from build123d import *

# Parameters (mm, degrees)
SKETCH1_R                = 17.45
SKETCH1_R_2              = 12.45
BOSS_EXTRUDE1_DEPTH      = 8
BOSS_EXTRUDE1_DEPTH_BACK = 25
SKETCH1_2_R              = 17.45
SKETCH1_2_R_2            = 12.45
BOSS_EXTRUDE3_DEPTH      = 18
SKETCH3_R                = 12.45
SKETCH3_R_2              = 8
BOSS_EXTRUDE4_DEPTH      = 3
SKETCH4_R                = 1
CUT_EXTRUDE1_DEPTH       = 10
SKETCH6_R                = 13.5
CUT_EXTRUDE2_DEPTH       = 40
SKETCH7_R                = 1
CUT_EXTRUDE3_DEPTH       = 21
CIRPATTERN1_COUNT        = 3
BOSS_EXTRUDE5_START      = -16.1
SKETCH8_R                = 20.25
SKETCH8_R_2              = 13.5
BOSS_EXTRUDE5_DEPTH      = 3
FILLET1_R                = 2
SKETCH9_W                = 226.458017819
SKETCH9_H                = 42.937005292
CUT_EXTRUDE4_DEPTH       = 34
CUT_EXTRUDE4_DEPTH_BACK  = 62
CUT_EXTRUDE5_START       = -1.9
CUT_EXTRUDE5_DEPTH       = 1.7
CUT_EXTRUDE5_DEPTH_BACK  = 1.3
SKETCH11_R               = 1
CUT_EXTRUDE6_DEPTH       = 3
CUT_EXTRUDE7_START       = -1.9
CUT_EXTRUDE7_DEPTH       = 1.7
SKETCH14_R               = 20.25
SKETCH14_R_2             = 1
SKETCH14_R_3             = 13.5
BOSS_EXTRUDE6_DEPTH      = 0.8


with BuildPart() as part:
    # Sketch1 → Boss-Extrude1 (new body, two sides)
    with BuildSketch(Plane(origin=(0, 0, 0), x_dir=(1, 0, 0), z_dir=(0, 1, 0))) as boss_extrude1_sk:
        Circle(SKETCH1_R)
        Circle(SKETCH1_R_2, mode=Mode.SUBTRACT)
    extrude(amount=BOSS_EXTRUDE1_DEPTH)
    extrude(boss_extrude1_sk.sketch, amount=-BOSS_EXTRUDE1_DEPTH_BACK)

    # Sketch1<2> → Boss-Extrude3 (add)
    with BuildSketch(Plane(origin=(0, 0, 0), x_dir=(1, 0, 0), z_dir=(0, 1, 0))):
        Circle(SKETCH1_2_R)
        Circle(SKETCH1_2_R_2, mode=Mode.SUBTRACT)
    extrude(amount=BOSS_EXTRUDE3_DEPTH)

    # Sketch3 → Boss-Extrude4 (add)
    with BuildSketch(Plane(origin=(0, 18, 0), x_dir=(1, 0, 0), z_dir=(0, 1, 0))):
        Circle(SKETCH3_R)
        Circle(SKETCH3_R_2, mode=Mode.SUBTRACT)
    extrude(amount=-BOSS_EXTRUDE4_DEPTH)

    # Sketch4 → Cut-Extrude1 (cut)
    with BuildSketch(Plane(origin=(0, 18, 0), x_dir=(1, 0, 0), z_dir=(0, 1, 0))):
        with Locations((9.526279442, 5.5)):
            Circle(SKETCH4_R)
        with Locations((-9.526279442, 5.5)):
            Circle(SKETCH4_R)
        with Locations((0, -11)):
            Circle(SKETCH4_R)
    extrude(amount=-CUT_EXTRUDE1_DEPTH, mode=Mode.SUBTRACT)

    # Sketch6 → Cut-Extrude2 (cut)
    with BuildSketch(Plane.XZ.offset(25)):
        Circle(SKETCH6_R)
    extrude(amount=-CUT_EXTRUDE2_DEPTH, mode=Mode.SUBTRACT)

    # Sketch7 → Cut-Extrude3 (cut)
    with BuildSketch(Plane.XY):
        with Locations((0, 12)):
            Circle(SKETCH7_R)
    cut_extrude3 = extrude(amount=-CUT_EXTRUDE3_DEPTH, mode=Mode.SUBTRACT)

    # CirPattern1: Cut-Extrude3 ×3 about axis
    cirpattern1_axis = Axis((0, 53.183766184, 0), (0, -1, 0))
    for i in range(1, CIRPATTERN1_COUNT):
        add(cut_extrude3.rotate(cirpattern1_axis, i * 360 / CIRPATTERN1_COUNT), mode=Mode.SUBTRACT)

    # Sketch8 → Boss-Extrude5 (add)
    with BuildSketch(Plane(origin=(0, 18, 0), x_dir=(1, 0, 0), z_dir=(0, 1, 0)).offset(BOSS_EXTRUDE5_START)):
        Circle(SKETCH8_R)
        Circle(SKETCH8_R_2, mode=Mode.SUBTRACT)
    extrude(amount=-BOSS_EXTRUDE5_DEPTH)

    # Fillet1
    fillet1_edges = [part.edges().sort_by_distance(p)[0] for p in [
        (-17.45, 18, 0),
    ]]
    fillet(fillet1_edges, radius=FILLET1_R)

    # Sketch9 → Cut-Extrude4 (cut, two sides)
    with BuildSketch(Plane(origin=(0, 0, 0), x_dir=(0, 0, -1), z_dir=(1, 0, 0))) as cut_extrude4_sk:
        with Locations((-4.854722567, -21.468502646)):
            Rectangle(SKETCH9_W, SKETCH9_H)
    extrude(amount=CUT_EXTRUDE4_DEPTH, mode=Mode.SUBTRACT)
    extrude(cut_extrude4_sk.sketch, amount=-CUT_EXTRUDE4_DEPTH_BACK, mode=Mode.SUBTRACT)

    # Sketch10 → Cut-Extrude5 (cut, two sides)
    with BuildSketch(Plane.XZ.offset(CUT_EXTRUDE5_START)) as cut_extrude5_sk:
        Polygon((12.701705922, -10), (15.011106999, -10), (16.165807537, -8), (15.011106999, -6), (12.701705922, -6), (11.547005384, -8), align=None)
        Polygon((-15.011106999, -6), (-16.165807537, -8), (-15.011106999, -10), (-12.701705922, -10), (-11.547005384, -8), (-12.701705922, -6), align=None)
        Polygon((-1.154700538, 18), (-2.309401077, 16), (-1.154700538, 14), (1.154700538, 14), (2.309401077, 16), (1.154700538, 18), align=None)
    extrude(amount=CUT_EXTRUDE5_DEPTH, mode=Mode.SUBTRACT)
    extrude(cut_extrude5_sk.sketch, amount=-CUT_EXTRUDE5_DEPTH_BACK, mode=Mode.SUBTRACT)

    # Sketch11 → Cut-Extrude6 (cut)
    with BuildSketch(Plane.XZ):
        with Locations((0, 16)):
            Circle(SKETCH11_R)
        with Locations((13.856406461, -8)):
            Circle(SKETCH11_R)
        with Locations((-13.856406461, -8)):
            Circle(SKETCH11_R)
    extrude(amount=-CUT_EXTRUDE6_DEPTH, mode=Mode.SUBTRACT)

    # Sketch13 → Cut-Extrude7 (cut)
    with BuildSketch(Plane.XZ.offset(CUT_EXTRUDE7_START)):
        Polygon((13.856406461, -12), (17.320508076, -6), (12.701705922, -6), (11.547005384, -8), align=None)
        Polygon((-17.064341974, -5.610617289), (-14.321704831, -11.972845004), (-11.562683328, -8.268640139), (-12.476895709, -6.147897568), align=None)
        Polygon((-3.464101615, 18), (-1.154700538, 14), (1.154700538, 14), (3.464101615, 18), align=None)
    extrude(amount=-CUT_EXTRUDE7_DEPTH, mode=Mode.SUBTRACT)

    # Sketch14 → Boss-Extrude6 (add)
    with BuildSketch(Plane.XZ):
        Circle(SKETCH14_R)
        with Locations((0, 16)):
            Circle(SKETCH14_R_2, mode=Mode.SUBTRACT)
        with Locations((13.856406461, -8)):
            Circle(SKETCH14_R_2, mode=Mode.SUBTRACT)
        with Locations((-13.856406461, -8)):
            Circle(SKETCH14_R_2, mode=Mode.SUBTRACT)
        Circle(SKETCH14_R_3, mode=Mode.SUBTRACT)
    extrude(amount=BOSS_EXTRUDE6_DEPTH)


solid = part.part
Work out the finished part from the listing and answer in its coordinate system (mm). A direction names the side the tool comes from. Coordinates: 2 decimals unless noted, no trailing zeros. Loops run counter-clockwise (first coordinate to the right, second up) from the corner with the lowest first, then second, coordinate; pieces in that order, holes last. Notation, with made-up numbers: M -12.75,45 L -1.75,45 A5 ccw -1.75,53 Z; hole C 44,38.25 d7. An arc over 180 degrees is marked long. Answer in a Markdown table with one row per item. Add a question column.
1. Consider L1, parallel to Z at x = 0, y = 0.15; L2, parallel to Z at x = 0, y = 15.75; L3, parallel to Z at x = 0, y = 10.75. Determine where each line is inside the solid, lowest interval first.
2. The mould has two halves that part along X. Classify faces 5 (the cylindrical face through (13.76, 11.39, 7.03)), 6 (the flat face through (-14, 3.6, -8)), 7 (the flat face through (-14.908, 2.738, -5.863)): pulls with the +X half, pulls with the -X half, needs draft (parallel to the pull), parting line crosses it, or undercut.
3. Find section B-B, the plane z = 0. Write down the section's boundary in (x, y), then the cut area to 3 significant figures.
4. A tool of negligible diameter and unlimited length cuts with its end or side. For faces 1 (the flat face through (-12.12, 1.35, -7.01)), 2 (the flat face through (6, 15, 6)), 3 (the flat face through (14, 3.6, -8)), 4 (the flat face through (0, 1, 18)), from which of +Z, -Z, +X, -X, +Y, -Y can it reach the whole face along a straight path? Write none if from no direction.
5. Find section A-A, the plane x = 0. State how many separate pieces and enclosed holes the cut face has, then the cut area to 3 significant figures.
6. Find section C-C, the plane y = 15.5. Write down the section's boundary in (x, z), then the cut area to 3 significant figures.
7. Flat-ended cylindrical pins translate along their axes: P1, Ø1.7, axis at x = 14.5, y = 2, coming from the -Z side; P2, Ø3, axis at x = 0, y = 12, coming from the +Z side; P3, Ø4, axis at x = -1.5, y = 9, coming from the -Z side; P4, Ø2, axis at x = -0.5, z = 5, coming from the -Y side. Find the tip coordinate at first contact, or state that the pin passes through.
8. Find section D-D, the plane y = 12. Write down the section's boundary in (x, z), then the cut area to 3 significant figures.
Reported:
| question | item | result |
|---|---|---|
| 1 | L1 | z = -20.25 to -13.5, 13.5 to 15, 17 to 20.25 |
| 1 | L2 | z = -17.45 to -8, 8 to 10, 12 to 17.45 |
| 1 | L3 | z = -17.45 to -13.5, 13.5 to 17.45 |
| 2 | face 5 | undercut |
| 2 | face 6 | needs draft |
| 2 | face 7 | pulls with the -X half |
| 3 | outline | M -20.25,-0.8 L -13.5,-0.8 L -13.5,15 L -8,15 L -8,18 L -15.45,18 A2 ccw -17.45,16 L -17.45,1.9 L -20.25,1.9 Z; M 8,15 L 13.5,15 L 13.5,-0.8 L 20.25,-0.8 L 20.25,1.9 L 17.45,1.9 L 17.45,16 A2 ccw 15.45,18 L 8,18 Z |
| 3 | area | 195 mm^2 |
| 4 | face 1 | none |
| 4 | face 2 | -Y |
| 4 | face 3 | +X |
| 4 | face 4 | +Y |
| 5 | separate pieces | 5 |
| 5 | enclosed holes | 0 |
| 5 | area | 166 mm^2 |
| 6 | outline | C 0,0 d34.9; hole C -9.53,-5.5 d2; hole C 0,0 d16; hole C 0,11 d2; hole C 9.53,-5.5 d2 |
| 6 | area | 746 mm^2 |
| 7 | P1 | stops at z = -14.95 |
| 7 | P2 | stops at z = 17.45 |
| 7 | P3 | stops at z = -17.45 |
| 7 | P4 | passes through |
| 8 | outline | M -15.59,7.84 A17.45 ccw -1,-17.42 L -1,-13.46 A13.5 cw -12.16,5.87 Z; M -14.59,9.58 L -11.16,7.6 A13.5 cw 11.16,7.6 L 14.59,9.58 A17.45 ccw Z; M 1,-17.42 A17.45 ccw 15.59,7.84 L 12.16,5.87 A13.5 cw 1,-13.46 Z |
| 8 | area | 360 mm^2 |
